Autodesk Inventor part; units mm, degrees
ref_plane "WorkPlane1" through (0, 0, 0) normal (0, 0, 1) x (1, 0, 0)
ref_plane "WorkPlane3" through (0, 0, -1.5748) normal (0, 0, 1) x (1, 0, 0)
ref_plane "Work Plane3" through (0, -6.1849, 0) normal (0, 1, 0) x (-1, 0, 0)
ref_plane "WorkPlane1" through (0, 0, 0) normal (0, 0, 1) x (1, 0, 0)
ref_plane "WorkPlane3" through (0, 0, -1.5748) normal (0, 0, 1) x (1, 0, 0)
ref_plane "Work Plane3" through (0, -6.1849, 0) normal (0, 1, 0) x (-1, 0, 0)
ref_plane "WorkPlane10" through (0, 6.1849, 0) normal (0, 1, 0) x (-1, 0, 0)
sketch "Sketch1" plane through (0, 0, 0) normal (0, 0, 1) x (1, 0, 0)
  point P0 (0, 0)
sketch "Sketch2" plane through (0, 0, 0) normal (0, 0, 1) x (1, 0, 0)
  circle A0 centre (0, 0) radius 6.1849
  dimension "d3" = 12.3698
extrude "Extrusion1" add sketch "Sketch2" against normal blind 1.5748
sketch "Sketch4" plane through (0, 0, 0) normal (0, 0, 1) x (1, 0, 0)
  circle A0 centre (0, 0) radius 6.1849
hole "Hole1" at (0, 0, 0) direction (0, 0, -1) diameter 6.4008 end through all
sketch "Sketch5" plane through (0, 6.1849, 0) normal (0, 1, 0) x (-1, 0, 0)
  line L0 (-0.0808, 0) -> (-0.4745, 0)
  line L1 (0.1969, -1.5748) -> (-0.0808, 0)
  line L2 (-0.1969, -1.5748) -> (0.1969, -1.5748)
  line L3 (-0.4745, 0) -> (-0.1969, -1.5748)
  line L4 (-3.2004, 0) -> (3.2004, 0) construction
  line L5 (6.1849, -1.5748) -> (-6.1849, -1.5748) construction
  line L6 (0, -3.048) -> (0, 0.508)
  dimension "d15" = 80
  dimension "d18" = 0.1968
  dimension "d19" = 0.1968
extrude "Extrusion2" cut sketch "Sketch5" against normal blind 6.1849
ref_plane "MSC_PT1" through (0, 0, 0) normal (0, 0, 1) x (1, 0, 0)
ref_plane "MSC_PT2" through (0, 0, -1.5748) normal (0, 0, -1) x (-1, 0, 0)
equation "\"d7\" = Diam1"
equation "\"d4\" = ParH"
equation "\"d18\" = 0.125 * ParH"
equation "\"d19\" = 0.125 * ParH"
equation "\"d16\" = 0.5 * Diam2"
equation "\"d3\" = Diam2"
equation "\"Diam2\" = 12.3698"
equation "\"ParH\" = 1.5748"
equation "\"Diam1\" = 6.4008"
equation "\"d20\" = 0.5 * Diam2"
properties part number "ANSI B18.21.1 - 0.25" material "Steel, Mild"
CAD build for the part. Positions are in the model's coordinates, mm. A direction names the side the tool comes from. Coordinates: 2 decimals unless noted, no trailing zeros. Order: outer loops, then holes, each group sorted by start corner. A loop starts at its lowest first (then second) coordinate and runs counter-clockwise, first axis right, second up.
Item 1: Drill centre lines: L1, parallel to X at y = 0.25, z = -1.45; L2, parallel to X at y = 5, z = -1.3. Where is each one in solid material? Low to high.
Check sheet entries:
L1: x = -6.18 to -3.19, 3.19 to 6.18
L2: x = -3.64 to -0.15, 0.25 to 3.64
Item 2: Band-saw the part on D-D on x = 5.25. List the corners of the cut face in (y, z), plus the area to 3 significant figures.
Check sheet entries:
outline: (-3.27, -1.57) - (3.27, -1.57) - (3.27, 0) - (-3.27, 0) - close
area: 10.3 mm2
Item 3: 3-axis set-ups, long thin cutter, end or side, ignore diameter. For faces 3 (the face through (0.338, 4.695, -0.776)), 4 (the face through (3, -3, -1.575)): which of +Z, -Z, +X, -X, +Y, -Y reach the whole face in a straight line?
Check sheet entries:
face 3: +Z, +Y
face 4: -Z, +X, -X, +Y, -Y
Item 4: Two-plate mould, pull along X, no slides. Class faces 1 (the face through (3, -3, 0)), 2 (the face through (-0.06, 4.71, -0.8)): +X half, -X half, draft (parallel to the pull), parting line (faces both ways), or undercut.
Check sheet entries:
face 1: draft
face 2: undercut
Item 5: Band-saw the part on B-B on z = -1.3. List the corners of the cut face in (x, y).
Check sheet entries:
outline: (-0.15, 3.2) - (-0.15, 6.18) arc R6.18 ccw (long way) to (0.25, 6.18) - (0.25, 3.19) arc R3.2 cw (long way) to start
Item 6: Band-saw the part on C-C on y = 2.25. List the corners of the cut face in (x, z).
Check sheet entries:
outline: (-5.76, -1.57) - (-2.28, -1.57) - (-2.28, 0) - (-5.76, 0) - close; (2.28, -1.57) - (5.76, -1.57) - (5.76, 0) - (2.28, 0) - close
Item 7: Band-saw the part on A-A on y = 0.25. List the corners of the cut face in (x, z).
Check sheet entries:
outline: (-6.18, -1.57) - (-3.19, -1.57) - (-3.19, 0) - (-6.18, 0) - close; (3.19, -1.57) - (6.18, -1.57) - (6.18, 0) - (3.19, 0) - close
